Design review of the part built by this model. Coordinates are the model's own, in mm. Give positions to 0.01 mm unless a question says otherwise; leave off trailing zeros. Order: outer loops, then holes, each group sorted by start corner. A loop starts at its lowest first (then second) coordinate and runs counter-clockwise, first axis right, second up.
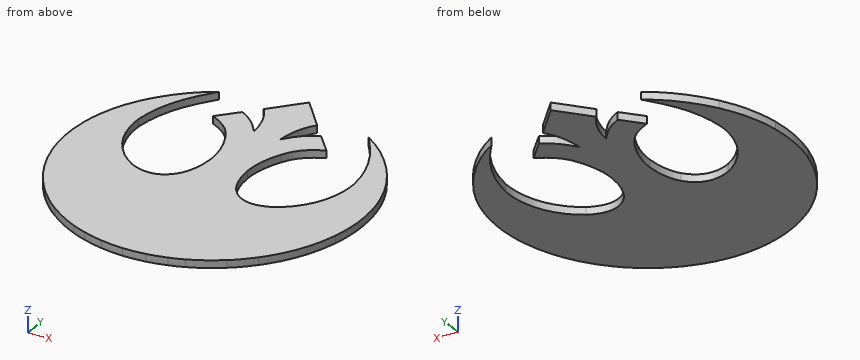
```python
from build123d import *

# Parameters (mm, degrees)
F1_DEPTH = 1


with BuildPart() as f1:
    # F0 (on Top) → F1 (new body)
    with BuildSketch(Plane.XY):
        with BuildLine():
            Line((3.579062, 15.997813), (0, 20.038363))
            Line((0, 20.038363), (-3.579062, 15.997813))
            add(Edge.make_bspline(
                [(-3.579062, 15.997813), (-2.214011, 14.396154), (-1.813596, 12.011866), (-1.777195, 11.029029)],
                knots=[0, 0, 0, 0, 5.285409, 5.285409, 5.285409, 5.285409], degree=3))
            add(Edge.make_bspline(
                [(-1.777195, 11.029029), (-2.742199, 12.312406), (-3.461874, 13.199826), (-5.253524, 14.141345)],
                knots=[0, 0, 0, 0, 4.66598, 4.66598, 4.66598, 4.66598], degree=3))
            Line((-5.253524, 14.141345), (-7.578195, 11.584778))
            add(Edge.make_bspline(
                [(-7.578195, 11.584778), (-4.584184, 10.274329), (-4.019963, 8.499763), (-3.728752, 7.999245)],
                knots=[0, 0, 0, 0, 5.260633, 5.260633, 5.260633, 5.260633], degree=3))
            add(Edge.make_bspline(
                [(-3.728752, 7.999245), (-2.700414, 5.997171), (-2.454705, 3.985996), (-2.500207, 2.802952)],
                knots=[0, 0, 0, 0, 5.339549, 5.339549, 5.339549, 5.339549], degree=3))
            add(Edge.make_bspline(
                [(-2.500207, 2.802952), (-2.573009, -0.072755), (-3.66505, -1.501508), (-3.819756, -1.747217)],
                knots=[0, 0, 0, 0, 4.737642, 4.737642, 4.737642, 4.737642], degree=3))
            add(Edge.make_bspline(
                [(-3.819756, -1.747217), (-4.365776, -2.402442), (-6.076639, -4.486419), (-9.525668, -2.739154)],
                knots=[0, 0, 0, 0, 5.791491, 5.791491, 5.791491, 5.791491], degree=3))
            add(Edge.make_bspline(
                [(-9.525668, -2.739154), (-10.633131, -2.132458), (-14.527799, 0.595101), (-14.390765, 6.540306)],
                knots=[0, 0, 0, 0, 10.477479, 10.477479, 10.477479, 10.477479], degree=3))
            add(Edge.make_bspline(
                [(-14.390765, 6.540306), (-13.981922, 11.711812), (-11.33765, 14.913963), (-9.977424, 16.72974)],
                knots=[0, 0, 0, 0, 11.104149, 11.104149, 11.104149, 11.104149], degree=3))
            add(Edge.make_bspline(
                [(-9.977424, 16.72974), (-12.846339, 15.039146), (-15.045267, 12.524201), (-16.459247, 10.330621)],
                knots=[0, 0, 0, 0, 9.10839, 9.10839, 9.10839, 9.10839], degree=3))
            add(Edge.make_bspline(
                [(-16.459247, 10.330621), (-17.365262, 8.871559), (-18.730281, 6.45445), (-19.280606, 2.758645)],
                knots=[0, 0, 0, 0, 8.080525, 8.080525, 8.080525, 8.080525], degree=3))
            add(Edge.make_bspline(
                [(-19.280606, 2.758645), (-19.793346, -0.917996), (-19.243021, -3.329711), (-18.94978, -4.69844)],
                knots=[0, 0, 0, 0, 7.46442, 7.46442, 7.46442, 7.46442], degree=3))
            add(Edge.make_bspline(
                [(-18.94978, -4.69844), (-17.765756, -9.674388), (-15.143621, -12.604054), (-14.20664, -13.638732)],
                knots=[0, 0, 0, 0, 10.120583, 10.120583, 10.120583, 10.120583], degree=3))
            add(Edge.make_bspline(
                [(-14.20664, -13.638732), (-13.403441, -14.51529), (-12.222866, -15.593206), (-11.504254, -16.068003)],
                knots=[0, 0, 0, 0, 3.633765, 3.633765, 3.633765, 3.633765], degree=3))
            add(Edge.make_bspline(
                [(-11.504254, -16.068003), (-9.972031, -17.249116), (-8.487965, -17.96635), (-7.431189, -18.424159)],
                knots=[0, 0, 0, 0, 4.705457, 4.705457, 4.705457, 4.705457], degree=3))
            add(Edge.make_bspline(
                [(-7.431189, -18.424159), (-6.675803, -18.752256), (-5.962383, -18.977345), (-5.542725, -19.107058)],
                knots=[0, 0, 0, 0, 2.008145, 2.008145, 2.008145, 2.008145], degree=3))
            add(Edge.make_bspline(
                [(-5.542725, -19.107058), (-4.604215, -19.412267), (-3.730562, -19.587761), (-2.978992, -19.709844)],
                knots=[0, 0, 0, 0, 2.633643, 2.633643, 2.633643, 2.633643], degree=3))
            add(Edge.make_bspline(
                [(-2.978992, -19.709844), (-2.017592, -19.87389), (-0.747171, -19.973081), (0, -19.961637)],
                knots=[0, 0, 0, 0, 2.989614, 2.989614, 2.989614, 2.989614], degree=3))
            add(Edge.make_bspline(
                [(2.978992, -19.709844), (2.017592, -19.87389), (0.747171, -19.973081), (0, -19.961637)],
                knots=[0, 0, 0, 0, 2.989614, 2.989614, 2.989614, 2.989614], degree=3))
            add(Edge.make_bspline(
                [(5.542725, -19.107058), (4.604215, -19.412267), (3.730562, -19.587761), (2.978992, -19.709844)],
                knots=[0, 0, 0, 0, 2.633643, 2.633643, 2.633643, 2.633643], degree=3))
            add(Edge.make_bspline(
                [(7.431189, -18.424159), (6.675803, -18.752256), (5.962383, -18.977345), (5.542725, -19.107058)],
                knots=[0, 0, 0, 0, 2.008145, 2.008145, 2.008145, 2.008145], degree=3))
            add(Edge.make_bspline(
                [(11.504254, -16.068003), (9.972031, -17.249116), (8.487965, -17.96635), (7.431189, -18.424159)],
                knots=[0, 0, 0, 0, 4.705457, 4.705457, 4.705457, 4.705457], degree=3))
            add(Edge.make_bspline(
                [(14.20664, -13.638732), (13.403441, -14.51529), (12.222866, -15.593206), (11.504254, -16.068003)],
                knots=[0, 0, 0, 0, 3.633765, 3.633765, 3.633765, 3.633765], degree=3))
            add(Edge.make_bspline(
                [(18.94978, -4.69844), (17.765756, -9.674388), (15.143621, -12.604054), (14.20664, -13.638732)],
                knots=[0, 0, 0, 0, 10.120583, 10.120583, 10.120583, 10.120583], degree=3))
            add(Edge.make_bspline(
                [(19.280606, 2.758645), (19.793346, -0.917996), (19.243021, -3.329711), (18.94978, -4.69844)],
                knots=[0, 0, 0, 0, 7.46442, 7.46442, 7.46442, 7.46442], degree=3))
            add(Edge.make_bspline(
                [(16.459247, 10.330621), (17.365262, 8.871559), (18.730281, 6.45445), (19.280606, 2.758645)],
                knots=[0, 0, 0, 0, 8.080525, 8.080525, 8.080525, 8.080525], degree=3))
            add(Edge.make_bspline(
                [(9.977424, 16.72974), (12.846339, 15.039146), (15.045267, 12.524201), (16.459247, 10.330621)],
                knots=[0, 0, 0, 0, 9.10839, 9.10839, 9.10839, 9.10839], degree=3))
            add(Edge.make_bspline(
                [(14.390765, 6.540306), (13.981922, 11.711812), (11.33765, 14.913963), (9.977424, 16.72974)],
                knots=[0, 0, 0, 0, 11.104149, 11.104149, 11.104149, 11.104149], degree=3))
            add(Edge.make_bspline(
                [(9.525668, -2.739154), (10.633131, -2.132458), (14.527799, 0.595101), (14.390765, 6.540306)],
                knots=[0, 0, 0, 0, 10.477479, 10.477479, 10.477479, 10.477479], degree=3))
            add(Edge.make_bspline(
                [(3.819756, -1.747217), (4.365776, -2.402442), (6.076639, -4.486419), (9.525668, -2.739154)],
                knots=[0, 0, 0, 0, 5.791491, 5.791491, 5.791491, 5.791491], degree=3))
            add(Edge.make_bspline(
                [(2.500207, 2.802952), (2.573009, -0.072755), (3.66505, -1.501508), (3.819756, -1.747217)],
                knots=[0, 0, 0, 0, 4.737642, 4.737642, 4.737642, 4.737642], degree=3))
            add(Edge.make_bspline(
                [(3.728752, 7.999245), (2.700414, 5.997171), (2.454705, 3.985996), (2.500207, 2.802952)],
                knots=[0, 0, 0, 0, 5.339549, 5.339549, 5.339549, 5.339549], degree=3))
            add(Edge.make_bspline(
                [(7.578195, 11.584778), (4.584184, 10.274329), (4.019963, 8.499763), (3.728752, 7.999245)],
                knots=[0, 0, 0, 0, 5.260633, 5.260633, 5.260633, 5.260633], degree=3))
            Line((7.578195, 11.584778), (5.253524, 14.141345))
            add(Edge.make_bspline(
                [(1.777195, 11.029029), (2.742199, 12.312406), (3.461874, 13.199826), (5.253524, 14.141345)],
                knots=[0, 0, 0, 0, 4.66598, 4.66598, 4.66598, 4.66598], degree=3))
            add(Edge.make_bspline(
                [(3.579062, 15.997813), (2.214011, 14.396154), (1.813596, 12.011866), (1.777195, 11.029029)],
                knots=[0, 0, 0, 0, 5.285409, 5.285409, 5.285409, 5.285409], degree=3))
        make_face()
    extrude(amount=F1_DEPTH)


solid = f1.part
```
1. Take a section at D-D (y = 18). State the section outline as (x, z) points.
Recorded:
outline: (-1.81, 0) - (1.81, 0) - (1.81, 1) - (-1.81, 1) - close
2. For line 1 along X through (y, z) = (3, 0.9); line 2 along X through (y, z) = (0, 0.85); line 3 along X through (y, z) = (12, 0.35), list the stretches that pass through material, from the lowest coordinate up.
Recorded:
line 1: x = -19.24 to -13.95, -2.5 to 2.5, 13.95 to 19.24
line 2: x = -19.49 to -12.5, -2.96 to 2.96, 12.5 to 19.49
line 3: x = -15.27 to -12.98, -7.2 to -2.54, -1.88 to 1.88, 2.54 to 7.2, 12.98 to 15.27
3. Take a section at A-A (y = 6). State how many separate pieces and enclosed holes the cut face has, then the cut area to 3 significant figures.
Recorded:
separate pieces: 3
enclosed holes: 0
area: 14.1 mm2
